Design review of the part shown in the three views and the two pictorial views. Dimensions are in mm from the part's minimum x, y and z. A direction names the side the tool comes from. Coordinates: 2 decimals unless noted, no trailing zeros. Loops run counter-clockwise (first coordinate to the right, second up) from the corner with the lowest first, then second, coordinate; pieces in that order, holes last. Notation, with made-up numbers: (4.25, 41) -> (14.25, 41) arc R18 cw to (14.25, 56) -> close; hole circle Ø5 at (-32, -26.5). An arc over 180 degrees is marked (long way). One line per item, written item: value. Start each with the question number.
1. Add section D-D on z = 44. Write out the cut boundary in (x, y) (1 decimal), plus the area to 3 significant figures.
2. Add section B-B on x = 20. Write out the cut boundary in (y, z).
3. Add section A-A on y = 10.5. Write out the cut boundary in (x, z), plus the area to 3 significant figures.
4. Machinability: for the marked faces 4, 5 and 6, which of the approach directions +Z, -Z, +X, -X, +Y, -Y give a long, thin tool a straight path to every point of the face, cutting with its end or side? Answer none if there is none.
5. Insertion check: pin 1 (4 mm diameter, centred on y = 17, z = 6.5, fed in from -X); pin 2 (0.9 mm diameter, centred on x = 43, z = 61, fed in from -Y); pin 3 (0.9 mm diameter, centred on y = 18, z = 60, fed in from +X). Each pin has a flat end and moves straight along its axis. Give the tip position at first contact, or say it passes through.
6. For probe 1 along Z at (x, y) = (32, 26); probe 2 along Y at (x, z) = (37, 39.5); probe 3 along Y at (x, z) = (12, 46.5), list the stretches that pass through material, from the lowest coordinate up.
7. Add section C-C on z = 22. Write out the cut boundary in (x, y), plus the area to 3 significant figures.
8. Draft analysis for pull direction Z (two halves, no side actions). For the marked faces 1, 2 and 3, state which applies: pulls with the +Z half, pulls with the -Z half, needs draft (parallel to the pull), parting line crosses it, or undercut.
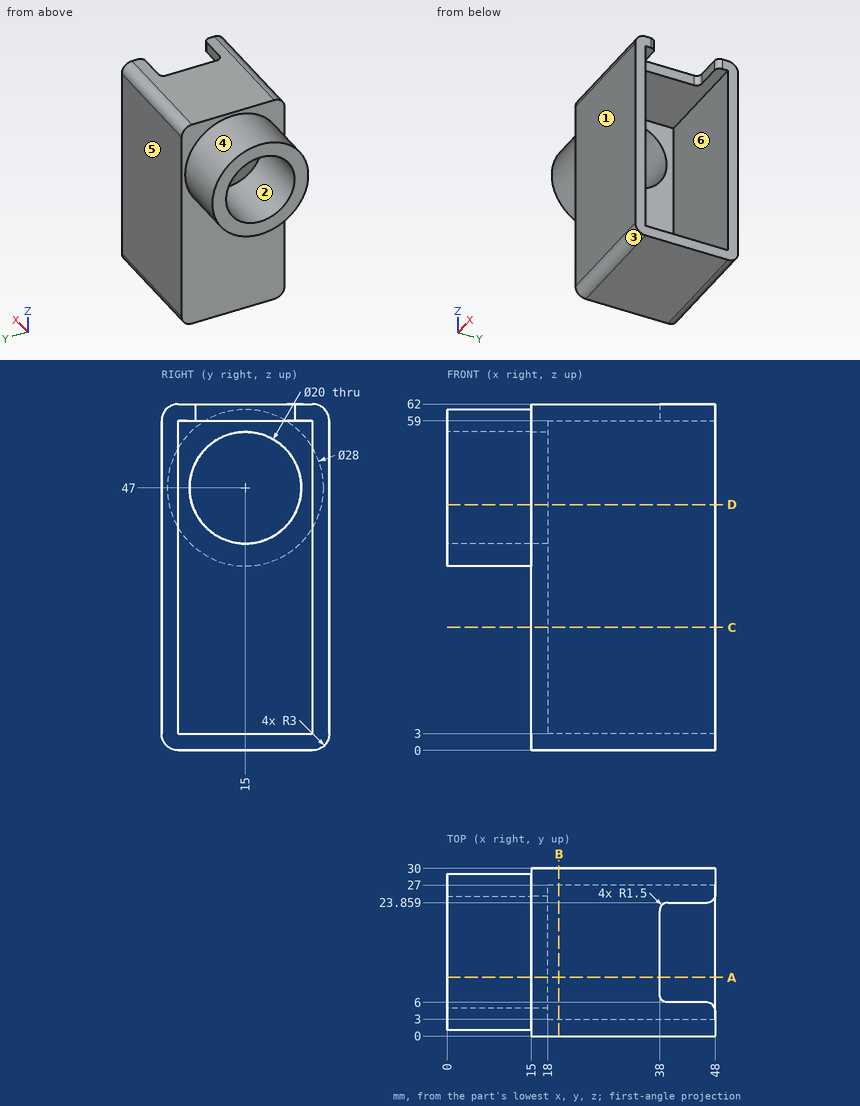
Worked answers:
1. outline: (0, 1.3) -> (15, 1.3) -> (15, 0) -> (48, 0) -> (48, 3) -> (18, 3) -> (18, 5.5) -> (0, 5.5) -> close; (0, 24.5) -> (18, 24.5) -> (18, 27) -> (48, 27) -> (48, 30) -> (15, 30) -> (15, 28.7) -> (0, 28.7) -> close
1. area: 337 mm²
2. outline: (0, 3) arc R3 ccw to (3, 0) -> (27, 0) arc R3 ccw to (30, 3) -> (30, 59) arc R3 ccw to (27, 62) -> (3, 62) arc R3 ccw to (0, 59) -> close; hole (3, 3) -> (27, 3) -> (27, 59) -> (3, 59) -> close
3. outline: (0, 33.74) -> (15, 33.74) -> (15, 0) -> (48, 0) -> (48, 3) -> (18, 3) -> (18, 38.07) -> (0, 38.07) -> close; (0, 55.93) -> (18, 55.93) -> (18, 59) -> (38, 59) -> (38, 62) -> (15, 62) -> (15, 60.26) -> (0, 60.26) -> close
3. area: 412 mm²
4. face 4: -X
4. face 5: +Z, -Z, +X, -X, +Y
4. face 6: +X
5. pin 1: stops at x = 15
5. pin 2: stops at y = 0.43
5. pin 3: stops at x = 38
6. probe 1: z = 0 to 3, 59 to 62
6. probe 2: y = 0 to 3, 27 to 30
6. probe 3: y = 1.01 to 5.01, 24.99 to 28.99
7. outline: (15, 0) -> (48, 0) -> (48, 3) -> (18, 3) -> (18, 27) -> (48, 27) -> (48, 30) -> (15, 30) -> close
7. area: 270 mm²
8. face 1: needs draft
8. face 2: undercut
8. face 3: pulls with the -Z half
